Autodesk Inventor part; units mm, degrees
ref_plane "YZ Plane" through (0, 0, 0) normal (1, 0, 0) x (0, 1, 0)
ref_plane "XZ Plane" through (0, 0, 0) normal (0, 1, 0) x (-1, 0, 0)
ref_plane "XY Plane" through (0, 0, 0) normal (0, 0, 1) x (1, 0, 0)
sketch "Sketch1" plane through (0, 0, 0) normal (0, 1, 0) x (-1, 0, 0)
  line L0 (-9.2075, -46.99) -> (9.2075, -46.99)
  line L1 (15.5575, -40.64) -> (15.5575, 46.99)
  line L2 (-15.5575, 46.99) -> (-15.5575, -40.64)
  line L3 (-15.5575, -46.99) -> (15.5575, 46.99) construction
  line L4 (15.5575, -46.99) -> (-15.5575, 46.99) construction
  circle A0 centre (0, -24.13) radius 2.54
  line L5 (8.89, -10.2337) -> (8.89, 27.8663)
  line L6 (-8.89, 27.8663) -> (-8.89, -10.2337)
  line L7 (-8.89, -10.2337) -> (8.89, 27.8663) construction
  line L8 (8.89, -10.2337) -> (-8.89, 27.8663) construction
  arc A1 (8.89, 27.8663) -> (-8.89, 27.8663) centre (0, 27.8663) ccw
  arc A2 (-8.89, -10.2337) -> (8.89, -10.2337) centre (0, -10.2337) ccw
  arc A3 (-8.89, 46.99) -> (8.89, 46.99) centre (0, 46.99) ccw
  line L9 (15.5575, 46.99) -> (8.89, 46.99)
  line L10 (-8.89, 46.99) -> (-15.5575, 46.99)
  arc A4 (9.2075, -46.99) -> (15.5575, -40.64) centre (9.2075, -40.64) ccw
  arc A5 (-15.5575, -40.64) -> (-9.2075, -46.99) centre (-9.2075, -40.64) ccw
  point P0 (0, 0)
  point P1 (0, 8.8163)
  dimension "d0" = 93.98
  dimension "d1" = 31.115
  dimension "d2" = 22.86
  dimension "d3" = 5.08
  dimension "d4" = 38.1
  dimension "d5" = 17.78
  dimension "d6" = 17.78
  dimension "d7" = 6.35
extrude "Extrusion1" add sketch "Sketch1" along normal blind 12.7
equation "\"d6\" = d5"
properties part number "Fixture_Slide_Lock_Plate"
Source: CAD feature listing. Evaluate the final solid. Frame: model axes, mm. A direction names the side the tool comes from. Coordinates: 2 decimals unless noted, no trailing zeros. Write each loop counter-clockwise with the first axis right and the second up, starting at its lowest first coordinate (ties: lowest second). Pieces come first, ordered by that corner, then holes. Notation, with made-up numbers: (-5.75, 40.25) - (50.25, 40.25) arc R19 ccw to (50.25, 54.25) - close; hole circle Ø4 at (-40, 39). An arc over 180 degrees is marked (long way). Answer as a JSON object with one key per item and string values.
Q1. Material intervals for line 1 (Z direction, x = 0, y = 4); line 2 (X direction, y = 2.5, z = -3.5); line 3 (Z direction, x = -2, y = 5), sorted ascending. Write a range as [from, to].
Ans:
{"line 1": "z = [-46.99, -26.67], [-21.59, -19.12], [36.76, 38.1]", "line 2": "x = [-15.56, -8.89], [8.89, 15.56]", "line 3": "z = [-46.99, -25.7], [-22.56, -18.9], [36.53, 38.33]"}
Q2. Section query D-D, the plane x = -7. Output: boundary loops of the cut face in (y, z).
Ans:
{"outline": "(0, -46.99) - (12.7, -46.99) - (12.7, -15.71) - (0, -15.71) - close; (0, 33.35) - (12.7, 33.35) - (12.7, 41.51) - (0, 41.51) - close"}
Q3. Section query C-C, the plane y = 1.5. Output: boundary loops of the cut face in (x, z).
Ans:
{"outline": "(-15.56, -40.64) arc R6.35 ccw to (-9.21, -46.99) - (9.21, -46.99) arc R6.35 ccw to (15.56, -40.64) - (15.56, 46.99) - (8.89, 46.99) arc R8.89 cw to (-8.89, 46.99) - (-15.56, 46.99) - close; hole (-8.89, -10.23) arc R8.89 ccw to (8.89, -10.23) - (8.89, 27.87) arc R8.89 ccw to (-8.89, 27.87) - close; hole circle Ø5.08 at (0, -24.13)"}
Q4. Section query A-A, the plane z = -24.13. Output: boundary loops of the cut face in (x, y), plus the area to 3 significant figures.
Ans:
{"outline": "(-15.56, 0) - (-2.54, 0) - (-2.54, 12.7) - (-15.56, 12.7) - close; (2.54, 0) - (15.56, 0) - (15.56, 12.7) - (2.54, 12.7) - close", "area": "331 mm2"}
Q5. Draft query along X for faces 1 (the flat face through (12, 6, 46.99)), 2 (the flat face through (-15.558, 6, 3)), 3 (the cylindrical face through (-0.195, 6.261, 38.102)). Return one class per face: released by +X, released by -X, zero draft, split by the parting line, or undercut.
Ans:
{"face 1": "zero draft", "face 2": "released by -X", "face 3": "undercut"}
Q6. Set-up query: faces 4 (the cylindrical face through (13.65, 6.26, -45.18)), 5 (the cylindrical face through (-0.2, 6.26, -19.12)). Return all of +Z, -Z, +X, -X, +Y, -Y with unobstructed straight access to the full face (end or side cutting, diameter ignored); none if empty.
Ans:
{"face 4": "-Z, +X, +Y, -Y", "face 5": "+Y, -Y"}
Q7. Section query B-B, the plane x = 0. Output: boundary loops of the cut face in (y, z), plus the area to 3 significant figures.
Ans:
{"outline": "(0, -46.99) - (12.7, -46.99) - (12.7, -26.67) - (0, -26.67) - close; (0, -21.59) - (12.7, -21.59) - (12.7, -19.12) - (0, -19.12) - close; (0, 36.76) - (12.7, 36.76) - (12.7, 38.1) - (0, 38.1) - close", "area": "306 mm2"}
